The listing builds one solid part. Answer for the finished solid, in the listing's coordinates (mm). Coordinates: 2 decimals unless noted, no trailing zeros. Order: outer loops, then holes, each group sorted by start corner. A loop starts at its lowest first (then second) coordinate and runs counter-clockwise, first axis right, second up. Notation, with made-up numbers: M -26,44.25 L -19,44.25 A8 ccw -19,51.25 Z; hole C 53.5,27 d8. An arc over 180 degrees is marked long. One line per item, written item: value. Start each with the question number.
Q1. The part is cut by section B-B on y = -7. Give the vertices of the cut face in (x, z), then the cut area to 3 significant figures.
Q2. Each of these flat-tipped pins is pushed along its axis until it touches: pin 1 Ø1 at (y, z) = (-72, 1) entering from -X; pin 2 Ø0.6 at (y, z) = (-50.5, 1.5) entering from +X. Where does it stop, or does it pass through?
Q3. Determine the mould class of faces 1 (the flat face through (45.46, -58.05, 0.99)), 2 (the cylindrical face through (23.5, -63.83, 1.01)), 3 (the flat face through (-48.06, 50.43, 0.99)) for opening direction Y: pulls with the +Y half, pulls with the -Y half, needs draft (parallel to the pull), parting line crosses it, or undercut.
Q4. The part is cut by section A-A on x = 3.5. Give the vertices of the cut face in (y, z), then the cut area to 3 significant figures.
Q5. The part is cut by section D-D on z = 1.6. Give the number of separate pieces and of enclosed holes in the cut face, then the cut area to 3 significant figures.
Q6. Straight lines are drawn through the part: line 1 along Y through (x, z) = (-25, 1.2); line 2 along Y through (x, z) = (35.5, 0.8); line 3 along Y through (x, z) = (-8, 1.65). For each, find the intervals that lie inside material, in ascending order. Write a range as [from, to].
Q7. The part is cut by section C-C on x = -25. Give the vertices of the cut face in (y, z).
```python
from build123d import *

# Parameters (mm, degrees)
SKETCH_1_W          = 100
SKETCH_1_H          = 132.2
SKETCH_1_W_2        = 15.2
SKETCH_1_H_2        = 2.2
SKETCH_1_W_3        = 2.2
SKETCH_1_H_3        = 15.2
SKETCH_1_H_4        = 20.2
EXTRUDE_1_DEPTH     = 2
CUT_EXTRUDE_1_DEPTH = 3
SKETCH_4_R          = 1.5
CUT_EXTRUDE_2_DEPTH = 10
SKETCH_2_R          = 0.5
CUT_EXTRUDE_3_DEPTH = 3
FILLET_1_R          = 1


with BuildPart() as part:
    # 草图1 → 凸台-拉伸1 (new body)
    with BuildSketch(Plane.XY):
        with Locations((0, -10)):
            Rectangle(SKETCH_1_W, SKETCH_1_H)
        with Locations((-30, -72)):
            Rectangle(SKETCH_1_W_2, SKETCH_1_H_2, mode=Mode.SUBTRACT)
        with Locations((-44, -48.4)):
            Rectangle(SKETCH_1_W_3, SKETCH_1_H_3, mode=Mode.SUBTRACT)
        with Locations((-44, -5.9)):
            Rectangle(SKETCH_1_W_3, SKETCH_1_H_4, mode=Mode.SUBTRACT)
        with Locations((0, -72)):
            Rectangle(SKETCH_1_W_2, SKETCH_1_H_2, mode=Mode.SUBTRACT)
        with Locations((30, -72)):
            Rectangle(SKETCH_1_W_2, SKETCH_1_H_2, mode=Mode.SUBTRACT)
        with Locations((44, -48.4)):
            Rectangle(SKETCH_1_W_3, SKETCH_1_H_3, mode=Mode.SUBTRACT)
        with Locations((44, -5.9)):
            Rectangle(SKETCH_1_W_3, SKETCH_1_H_4, mode=Mode.SUBTRACT)
        with Locations((-44, 34.1)):
            Rectangle(SKETCH_1_W_3, SKETCH_1_H_4, mode=Mode.SUBTRACT)
        with Locations((44, 34.1)):
            Rectangle(SKETCH_1_W_3, SKETCH_1_H_4, mode=Mode.SUBTRACT)
    extrude(amount=EXTRUDE_1_DEPTH)

    # 草图3 → 切除-拉伸1 (cut, through all)
    with BuildSketch(Plane(origin=(0, 0, 0), x_dir=(-1, 0, 0), z_dir=(0, 0, -1))):
        Polygon((50, 45.1), (50, 56.1), (45.996327423, 56.1), align=None)
        Polygon((-50, 45.1), (-50, 56.1), (-45.996327423, 56.1), align=None)
        Polygon((-50, -41.1), (-40.621778265, -76.1), (-50, -76.1), align=None)
        Polygon((40.621778265, -76.1), (50, -76.1), (50, -41.1), align=None)
    extrude(amount=-CUT_EXTRUDE_1_DEPTH, mode=Mode.SUBTRACT)

    # 草图4 → 切除-拉伸2 (cut)
    with BuildSketch(Plane.XY.offset(2)):
        with Locations((-25, -3.9)):
            Circle(SKETCH_4_R)
        with Locations((25, -3.9)):
            Circle(SKETCH_4_R)
        with Locations((-25, -33.9)):
            Circle(SKETCH_4_R)
        with Locations((25, -33.9)):
            Circle(SKETCH_4_R)
        with Locations((25, -63.9)):
            Circle(SKETCH_4_R)
        with Locations((-25, -63.9)):
            Circle(SKETCH_4_R)
    extrude(amount=-CUT_EXTRUDE_2_DEPTH, mode=Mode.SUBTRACT)

    # 草图2 → 切除-拉伸3 (cut, through all)
    with BuildSketch(Plane.XY.offset(2)):
        with Locations((-45.1, 44.2)):
            Circle(SKETCH_2_R)
        with Locations((-42.9, 44.2)):
            Circle(SKETCH_2_R)
        with Locations((-45.1, 24)):
            Circle(SKETCH_2_R)
        with Locations((-42.9, 24)):
            Circle(SKETCH_2_R)
        with Locations((-45.1, 4.2)):
            Circle(SKETCH_2_R)
        with Locations((-42.9, 4.2)):
            Circle(SKETCH_2_R)
        with Locations((-45.1, -16)):
            Circle(SKETCH_2_R)
        with Locations((-42.9, -16)):
            Circle(SKETCH_2_R)
        with Locations((-45.1, -40.8)):
            Circle(SKETCH_2_R)
        with Locations((-42.9, -40.8)):
            Circle(SKETCH_2_R)
        with Locations((-45.1, -56)):
            Circle(SKETCH_2_R)
        with Locations((-42.9, -56)):
            Circle(SKETCH_2_R)
        with Locations((-37.6, -70.9)):
            Circle(SKETCH_2_R)
        with Locations((-37.6, -73.1)):
            Circle(SKETCH_2_R)
        with Locations((-22.4, -70.9)):
            Circle(SKETCH_2_R)
        with Locations((-22.4, -73.1)):
            Circle(SKETCH_2_R)
        with Locations((-7.6, -70.9)):
            Circle(SKETCH_2_R)
        with Locations((-7.6, -73.1)):
            Circle(SKETCH_2_R)
        with Locations((7.6, -73.1)):
            Circle(SKETCH_2_R)
        with Locations((7.6, -70.9)):
            Circle(SKETCH_2_R)
        with Locations((22.4, -73.1)):
            Circle(SKETCH_2_R)
        with Locations((22.4, -70.9)):
            Circle(SKETCH_2_R)
        with Locations((37.6, -73.1)):
            Circle(SKETCH_2_R)
        with Locations((37.6, -70.9)):
            Circle(SKETCH_2_R)
        with Locations((42.9, -56)):
            Circle(SKETCH_2_R)
        with Locations((45.1, -56)):
            Circle(SKETCH_2_R)
        with Locations((42.9, -40.8)):
            Circle(SKETCH_2_R)
        with Locations((45.1, -40.8)):
            Circle(SKETCH_2_R)
        with Locations((42.9, -16)):
            Circle(SKETCH_2_R)
        with Locations((45.1, -16)):
            Circle(SKETCH_2_R)
        with Locations((42.9, 4.2)):
            Circle(SKETCH_2_R)
        with Locations((45.1, 4.2)):
            Circle(SKETCH_2_R)
        with Locations((42.9, 24)):
            Circle(SKETCH_2_R)
        with Locations((45.1, 24)):
            Circle(SKETCH_2_R)
        with Locations((42.9, 44.2)):
            Circle(SKETCH_2_R)
        with Locations((45.1, 44.2)):
            Circle(SKETCH_2_R)
    extrude(amount=-CUT_EXTRUDE_3_DEPTH, mode=Mode.SUBTRACT)

    # 圆角1
    fillet_1_edges = [part.edges().sort_by_distance(p)[0] for p in [
        (-50, 45.1, 1),
        (-45.996327423, 56.1, 1),
        (50, -41.1, 1),
        (40.621778265, -76.1, 1),
        (-40.621778265, -76.1, 1),
        (-50, -41.1, 1),
        (45.996327423, 56.1, 1),
        (50, 45.1, 1),
    ]]
    fillet(fillet_1_edges, radius=FILLET_1_R)


solid = part.part
```
Output:
1. outline: M -50,0 L -45.1,0 L -45.1,2 L -50,2 Z; M -42.9,0 L 42.9,0 L 42.9,2 L -42.9,2 Z; M 45.1,0 L 50,0 L 50,2 L 45.1,2 Z
1. area: 191 mm^2
2. pin 1: stops at x = -41.85
2. pin 2: stops at x = 47.56
3. face 1: pulls with the -Y half
3. face 2: undercut
3. face 3: pulls with the +Y half
4. outline: M -76.1,0 L -73.1,0 L -73.1,2 L -76.1,2 Z; M -70.9,0 L 56.1,0 L 56.1,2 L -70.9,2 Z
4. area: 260 mm^2
5. separate pieces: 1
5. enclosed holes: 15
5. area: 12,400 mm^2
6. line 1: y = [-76.1, -73.1], [-70.9, -65.4], [-62.4, -35.4], [-32.4, -5.4], [-2.4, 56.1]
6. line 2: y = [-76.1, -73.1], [-70.9, 56.1]
6. line 3: y = [-76.1, -73.4], [-72.8, -71.2], [-70.6, 56.1]
7. outline: M -76.1,0 L -73.1,0 L -73.1,2 L -76.1,2 Z; M -70.9,0 L -65.4,0 L -65.4,2 L -70.9,2 Z; M -62.4,0 L -35.4,0 L -35.4,2 L -62.4,2 Z; M -32.4,0 L -5.4,0 L -5.4,2 L -32.4,2 Z; M -2.4,0 L 56.1,0 L 56.1,2 L -2.4,2 Z
